```python
from build123d import *

# Parameters (mm, degrees)
F7_DEPTH = 4


with BuildPart() as f5:
    # F2 (on Top) → F5 section 0
    with BuildSketch(Plane.XY):
        with BuildLine():
            add(Edge.make_bspline(
                [(-42.1898663044, 0), (-20.095104951, 6.3461639408), (16.4689935563, 16.848280699), (33.6635201253, 4.7769359586), (40.4678285122, 0)],
                knots=[0, 0, 0, 0, 0.6042747464, 1, 1, 1, 1], degree=3))
            Line((-42.1898663044, 0), (40.4678285122, 0))
        make_face()
    # F4 (on offset) → F5 section 1
    with BuildSketch(Plane.XY.offset(270)):
        with BuildLine():
            add(Edge.make_bspline(
                [(-42.1898663044, 0), (-20.9629036859, 6.7867963825), (110.2383227264, 31.3871603736), (189.1823338107, 6.6216905533), (197.8101336956, 0)],
                knots=[0, 0, 0, 0, 0.5699540347, 1, 1, 1, 1], degree=3))
            Line((-42.1898663044, 0), (197.8101336956, 0))
        make_face()
    loft()

    # F6 (on face) → F7 (join)
    with BuildSketch(Plane(origin=(0, 0, 0), x_dir=(1, 0, 0), z_dir=(0, 0, -1))):
        with BuildLine():
            add(Edge.make_bspline(
                [(40.4678285122, 0), (37.8826727608, -14.0204940933), (45.9325195, -67.5326493396), (-22.4150604159, -60.996185377), (-42.1898663044, -60)],
                knots=[0, 0, 0, 0, 0.4587258224, 1, 1, 1, 1], degree=3))
            Line((40.4678285122, 0), (-42.1898663044, 0))
            Line((-42.1898663044, 0), (-42.1898663044, -60))
        make_face()
    extrude(amount=F7_DEPTH)

    # F8: F5 across face


with BuildPart() as f5_1:
    add(f5.part)
    add(f5.part.mirror(Plane(origin=(85.8641490602, 7.5856772393, 270), x_dir=(1, 0, 0), z_dir=(0, 0, 1))))


solid = f5_1.part
```
Could you check a few things on this model? Use its own coordinates, in mm. Round coordinates to 2 decimals unless told otherwise and drop trailing zeros. Put each result on its own line as item: value.
Q1. I need wall thicknesses on probe 1 along Z at (x, y) = (14, 44); probe 2 along Y at (x, z) = (-20, 503); probe 3 along Y at (x, z) = (39.5, 272). Which ranges of each line are inside material? Lowest first, please.
Check result:
probe 1: -4 to 0, 540 to 544
probe 2: 0 to 5.94
probe 3: 0 to 15.1
Q2. Thinking about a two-plate mould opening in Z: for faces 1 (the face through (-7, 33, 540)), 2 (the face through (53, 0, 266)), 3 (the face through (-7, 26, -4)), which applies, released by +Z, released by -Z, zero draft, split by the parting line, or undercut?
Check result:
face 1: undercut
face 2: zero draft
face 3: released by -Z
Q3. For pin 1 (12 mm diameter, centred on y = 10.5, z = 444, fed in from +X), with a flat end and sliding along its axis, tell me the tip position at first contact or that it passes through.
Check result:
pin 1: x = 89.21
